from build123d import *

# Parameters (mm, degrees)
SKETCH1_W           = 7
SKETCH1_H           = 20
SKETCH1_R           = 2
BOSS_EXTRUDE1_DEPTH = 3.5
FILLET1_R           = 3.5
FILLET2_R           = 0.5


with BuildPart() as part:
    # Sketch1 → Boss-Extrude1 (new, symmetric)
    with BuildSketch(Plane.XY):
        with Locations((0, -5)):
            Rectangle(SKETCH1_W, SKETCH1_H)
        Circle(SKETCH1_R, mode=Mode.SUBTRACT)
    extrude(amount=BOSS_EXTRUDE1_DEPTH, both=True)

    # Fillet1
    # the kernel refuses this fillet: 3.5 mm, written as the material it takes off along each edge
    with BuildSketch(Plane(origin=(-12.25, 5, 3.5), x_dir=(0, 0, -1), z_dir=(1, 0, 0)), Plane(origin=(-3.5, 5, -12.25), x_dir=(1, 0, 0), z_dir=(0, 0, 1)), Plane(origin=(3.5, 5, 12.25), x_dir=(-1, 0, 0), z_dir=(0, 0, -1))) as fillet1_piece_1:
        with BuildLine():
            CenterArc((FILLET1_R, -FILLET1_R), FILLET1_R, 90, 90)
            Line((0, -FILLET1_R), (0, 0))
            Line((0, 0), (FILLET1_R, 0))
        make_face()
    extrude(amount=24.5, mode=Mode.SUBTRACT)
    with BuildSketch(Plane(origin=(-12.25, 5, -3.5), x_dir=(0, 0, 1), z_dir=(1, 0, 0))) as fillet1_piece_2:
        with BuildLine():
            CenterArc((FILLET1_R, FILLET1_R), FILLET1_R, 180, 90)
            Line((0, FILLET1_R), (0, 0))
            Line((0, 0), (FILLET1_R, 0))
        make_face()
    extrude(amount=24.5, mode=Mode.SUBTRACT)

    # Fillet2
    fillet2_edges = [part.edges().sort_by_distance(p)[0] for p in [
        (3.5, -6.75, 3.5),
        (-3.5, -6.75, 3.5),
        (-3.5, -6.75, -3.5),
        (-2.261171176, 4.171536059, 2.261171176),
        (-2.261171176, 4.171536059, -2.261171176),
        (2.261171176, 4.171536059, 2.261171176),
        (2.261171176, 4.171536059, -2.261171176),
        (3.5, -6.75, -3.5),
        (0, -15, -3.5),
        (0, -15, 3.5),
        (3.5, -15, 0),
        (-3.5, -15, 0),
    ]]
    fillet(fillet2_edges, radius=FILLET2_R)


solid = part.part
Geometry: final body of the model. Coordinates: model frame, mm. Give positions to 0.01 mm unless a question says otherwise; leave off trailing zeros. Order: outer loops, then holes, each group sorted by start corner. A loop starts at its lowest first (then second) coordinate and runs counter-clockwise, first axis right, second up. Notation, with made-up numbers: (-37.5, 32) -> (-9.5, 32) arc R30 cw to (-9.5, 58) -> close; hole circle Ø6 at (63, 31.5). An arc over 180 degrees is marked (long way). Put each result on its own line as item: value.
Q1. Section A-A, the plane y = 0. Return loops of the section in (x, z).
Here are the results:
outline: (-3.5, -3) arc R0.5 ccw to (-3, -3.5) -> (-2, -3.5) -> (-2, 3.5) -> (-3, 3.5) arc R0.5 ccw to (-3.5, 3) -> close; (2, -3.5) -> (3, -3.5) arc R0.5 ccw to (3.5, -3) -> (3.5, 3) arc R0.5 ccw to (3, 3.5) -> (2, 3.5) -> close
Q2. Material intervals for L1, parallel to X at y = 0, z = 0.5; L2, parallel to Y at x = 0.25, z = 1; L3, parallel to Y at x = 0, z = -1.5, sorted ascending.
Here are the results:
L1: x = -3.5 to -2, 2 to 3.5
L2: y = -15 to -1.98, 1.98 to 4.85
L3: y = -15 to -2, 2 to 4.66
Q3. Pin query (flat end, axial travel): pin 1 (1.5 mm diameter, centred on x = 0.5, y = 2.5, fed in from -Z). Return the tip coordinate at first contact, or that it passes through.
Here are the results:
pin 1: stops at z = -3.49
Q4. Draft query along X for faces 1 (the face through (0, -6, -3.5)), 2 (the face through (0, -2, 0)), 3 (the face through (2.889, 3.476, -0.042)), 4 (the face through (-2.845, 3.539, -0.042)). Return one class per face: released by +X, released by -X, zero draft, split by the parting line, or undercut.
Here are the results:
face 1: zero draft
face 2: undercut
face 3: released by +X
face 4: released by -X
